Answer from the drawing. Dimensions are ordinates in mm from the lowest x, y and z of the part. A direction names the side the tool comes from. Give positions to 0.01 mm unless a question says otherwise; leave off trailing zeros. Write each loop counter-clockwise with the first axis right and the second up, starting at its lowest first coordinate (ties: lowest second). Pieces come first, ordered by that corner, then holes. Notation, with made-up numbers: (43, 7.5) -> (61, 7.5) arc R22 cw to (61, 18.5) -> close; hole circle Ø8 at (81.5, 33). An arc over 180 degrees is marked (long way). Use a Markdown table: item, result. Add a question column.
Q1. Section D-D, the plane z = 25 is taken. Give the vertices of the cut face in (x, y), plus the area to 3 significant figures.
Q2. Consider line 1 (Y direction, x = 39, z = 50); line 2 (Y direction, x = 32, z = 61); line 3 (Z direction, x = 65, y = 21). Determine where each line is inside the solid, lowest interval first.
Q3. Section A-A, the plane z = 50 is taken. Give the vertices of the cut face in (x, y), plus the area to 3 significant figures.
Q4. For the marked faces 1 and 2, determine the directions among +Z, -Z, +X, -X, +Y, -Y from which every point of the face is accessible in a straight line to the end or side of a thin tool.
Q5. Section C-C, the plane y = 160 is taken. Give the vertices of the cut face in (x, z), plus the area to 3 significant figures.
Q6. For a pull along Z with two mould halves and no side action, classify the marked faces 3, 4, 5 and 6 as pulls with the +Z half, pulls with the -Z half, needs draft (parallel to the pull), parting line crosses it, or undercut.
Q7. Section B-B, the plane x = 76.5 is taken. Give the vertices of the cut face in (y, z), plus the area to 3 significant figures.
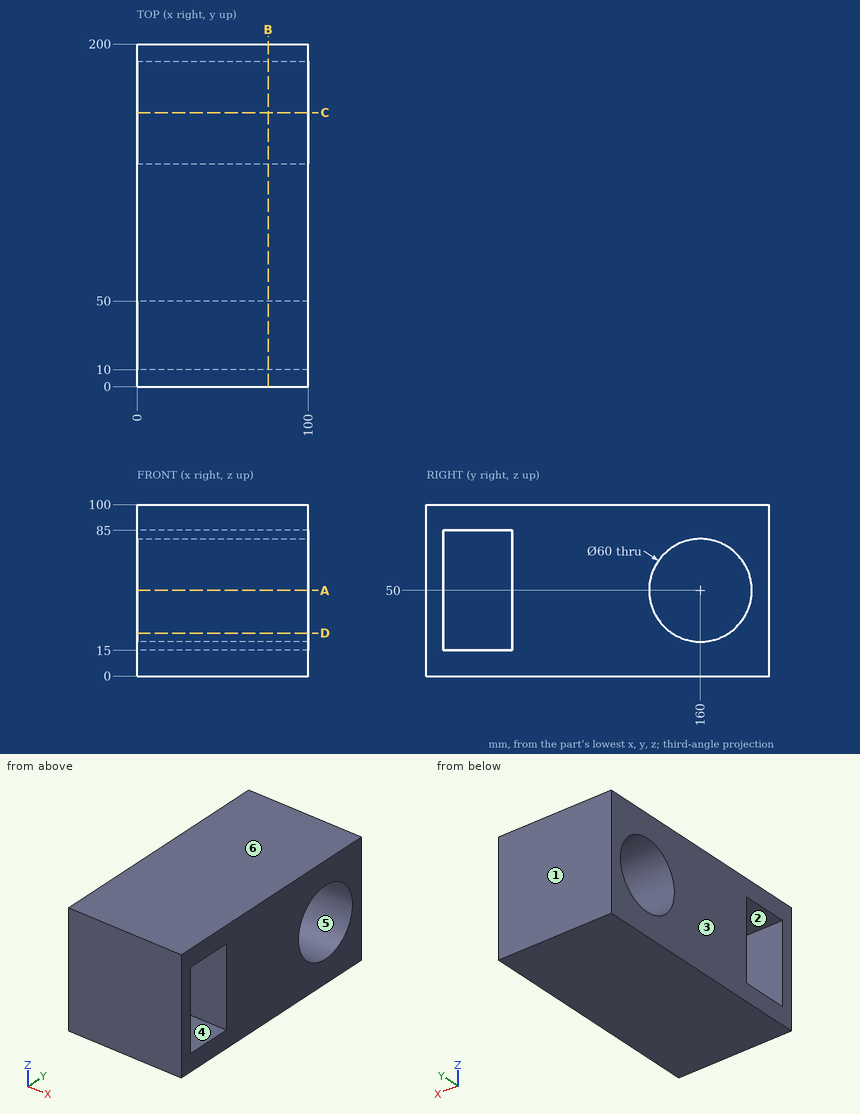
Result set:
| question | item | result |
|---|---|---|
| 1 | outline | (0, 0) -> (100, 0) -> (100, 10) -> (0, 10) -> close; (0, 50) -> (100, 50) -> (100, 143.42) -> (0, 143.42) -> close; (0, 176.58) -> (100, 176.58) -> (100, 200) -> (0, 200) -> close |
| 1 | area | 12,700 mm2 |
| 2 | line 1 | y = 0 to 10, 50 to 130, 190 to 200 |
| 2 | line 2 | y = 0 to 10, 50 to 132.09, 187.91 to 200 |
| 2 | line 3 | z = 0 to 15, 85 to 100 |
| 3 | outline | (0, 0) -> (100, 0) -> (100, 10) -> (0, 10) -> close; (0, 50) -> (100, 50) -> (100, 130) -> (0, 130) -> close; (0, 190) -> (100, 190) -> (100, 200) -> (0, 200) -> close |
| 3 | area | 10,000 mm2 |
| 4 | face 1 | +Z, -Z, +X, -X, +Y |
| 4 | face 2 | +X, -X |
| 5 | outline | (0, 0) -> (100, 0) -> (100, 20) -> (0, 20) -> close; (0, 80) -> (100, 80) -> (100, 100) -> (0, 100) -> close |
| 5 | area | 4,000 mm2 |
| 6 | face 3 | needs draft |
| 6 | face 4 | undercut |
| 6 | face 5 | undercut |
| 6 | face 6 | pulls with the +Z half |
| 7 | outline | (0, 0) -> (200, 0) -> (200, 100) -> (0, 100) -> close; hole (10, 15) -> (50, 15) -> (50, 85) -> (10, 85) -> close; hole circle Ø60 at (160, 50) |
| 7 | area | 14,400 mm2 |
